Geometry: final body of the model. Coordinates: model frame, mm. Round coordinates to 2 decimals unless told otherwise and drop trailing zeros. Order: outer loops, then holes, each group sorted by start corner. A loop starts at its lowest first (then second) coordinate and runs counter-clockwise, first axis right, second up. Notation, with made-up numbers: M 55,-27.5 L 96,-27.5 A17 ccw 96,-19.5 Z; hole C 78,-3 d8. An arc over 180 degrees is marked long. Return JSON: item names as keys, results as strings. Group by question number.
Q1. Cut plane A-A on z = -46.5. Output: boundary loops of the cut face in (x, y), and give its area (3 significant figures).
Q2. Contact query for flat-ended pins moving along their axis: pin 1 (3 mm diameter, centred on x = -2.5, z = 11, fed in from +Y); pin 2 (3 mm diameter, centred on x = -56, z = -91, fed in from +Y). Output: stop coordinate, or through.
Q3. Cut plane B-B on y = 1.4. Count the separate pieces of the cut face and the enclosed holes in it, and give its area (3 significant figures).
Q4. Ray query, probe 1 along X at (y, z) = (1.7, -58.5); probe 2 along X at (y, z) = (2.4, -9) (3 decimals); probe 3 along Z at (x, y) = (-91, 2.4). Return the intervals inside material, ascending.
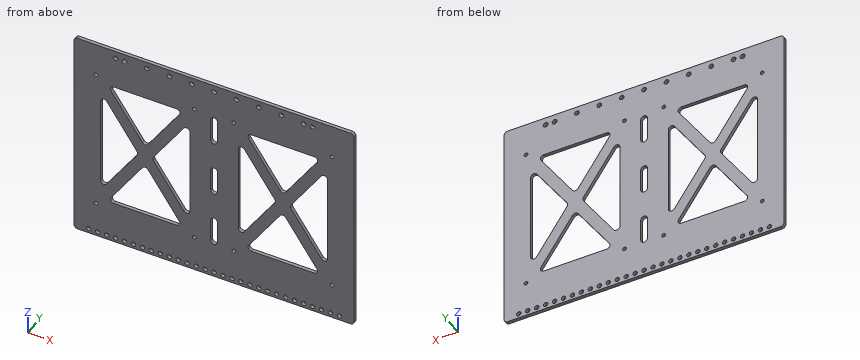
```python
from build123d import *

# Parameters (mm, degrees)
SKETCH_1_W               = 250
SKETCH_1_H               = 190
EXTRUDE_1_DEPTH          = 3
CUT_EXTRUDE_1_DEPTH      = 158.031843904
CUT_EXTRUDE_1_DEPTH_BACK = 158.031843904
SKETCH_3_R               = 2.15
CUT_EXTRUDE_2_DEPTH      = 158.031843904
SKETCH_4_R               = 2.1
CUT_EXTRUDE_3_DEPTH      = 158.031843904
CUT_EXTRUDE_4_DEPTH      = 158.031843904
FILLET_1_R               = 3
CUT_EXTRUDE_5_DEPTH      = 158.031843904


with BuildPart() as part:
    # 草图1 → 凸台-拉伸1 (new body)
    with BuildSketch(Plane(origin=(0, 0, 0), x_dir=(1, 0, 0), z_dir=(0, 1, 0))):
        Rectangle(SKETCH_1_W, SKETCH_1_H)
    extrude(amount=EXTRUDE_1_DEPTH)

    # 草图2 → 切除-拉伸1 (cut, two sides: drawn at the far end of the back side and taken through both)
    with BuildSketch(Plane.XZ.offset(-CUT_EXTRUDE_1_DEPTH_BACK)):
        with BuildLine():
            ThreePointArc((56, -93), (58, -91), (56, -89))
            ThreePointArc((56, -89), (54, -91), (56, -93))
        make_face()
        with BuildLine():
            ThreePointArc((-112, -93), (-110, -91), (-112, -89))
            ThreePointArc((-112, -89), (-114, -91), (-112, -93))
        make_face()
        with BuildLine():
            ThreePointArc((-104, -93), (-102, -91), (-104, -89))
            ThreePointArc((-104, -89), (-106, -91), (-104, -93))
        make_face()
        with BuildLine():
            ThreePointArc((-96, -93), (-94, -91), (-96, -89))
            ThreePointArc((-96, -89), (-98, -91), (-96, -93))
        make_face()
        with BuildLine():
            ThreePointArc((-88, -93), (-86, -91), (-88, -89))
            ThreePointArc((-88, -89), (-90, -91), (-88, -93))
        make_face()
        with BuildLine():
            ThreePointArc((-48, -93), (-46, -91), (-48, -89))
            ThreePointArc((-48, -89), (-50, -91), (-48, -93))
        make_face()
        with BuildLine():
            ThreePointArc((-80, -93), (-78, -91), (-80, -89))
            ThreePointArc((-80, -89), (-82, -91), (-80, -93))
        make_face()
        with BuildLine():
            ThreePointArc((-72, -93), (-70, -91), (-72, -89))
            ThreePointArc((-72, -89), (-74, -91), (-72, -93))
        make_face()
        with BuildLine():
            ThreePointArc((-64, -93), (-62, -91), (-64, -89))
            ThreePointArc((-64, -89), (-66, -91), (-64, -93))
        make_face()
        with BuildLine():
            ThreePointArc((-56, -93), (-54, -91), (-56, -89))
            ThreePointArc((-56, -89), (-58, -91), (-56, -93))
        make_face()
        with BuildLine():
            ThreePointArc((64, -93), (66, -91), (64, -89))
            ThreePointArc((64, -89), (62, -91), (64, -93))
        make_face()
        with BuildLine():
            ThreePointArc((72, -93), (74, -91), (72, -89))
            ThreePointArc((72, -89), (70, -91), (72, -93))
        make_face()
        with BuildLine():
            ThreePointArc((80, -93), (82, -91), (80, -89))
            ThreePointArc((80, -89), (78, -91), (80, -93))
        make_face()
        with BuildLine():
            ThreePointArc((88, -93), (90, -91), (88, -89))
            ThreePointArc((88, -89), (86, -91), (88, -93))
        make_face()
        with BuildLine():
            ThreePointArc((96, -93), (98, -91), (96, -89))
            ThreePointArc((96, -89), (94, -91), (96, -93))
        make_face()
        with BuildLine():
            ThreePointArc((104, -93), (106, -91), (104, -89))
            ThreePointArc((104, -89), (102, -91), (104, -93))
        make_face()
        with BuildLine():
            ThreePointArc((112, -93), (114, -91), (112, -89))
            ThreePointArc((112, -89), (110, -91), (112, -93))
        make_face()
        with BuildLine():
            ThreePointArc((32, -93), (34, -91), (32, -89))
            ThreePointArc((32, -89), (30, -91), (32, -93))
        make_face()
        with BuildLine():
            ThreePointArc((24, -93), (26, -91), (24, -89))
            ThreePointArc((24, -89), (22, -91), (24, -93))
        make_face()
        with BuildLine():
            ThreePointArc((16, -93), (18, -91), (16, -89))
            ThreePointArc((16, -89), (14, -91), (16, -93))
        make_face()
        with BuildLine():
            ThreePointArc((8, -93), (10, -91), (8, -89))
            ThreePointArc((8, -89), (6, -91), (8, -93))
        make_face()
        with BuildLine():
            ThreePointArc((0, -93), (2, -91), (0, -89))
            ThreePointArc((0, -89), (-2, -91), (0, -93))
        make_face()
        with BuildLine():
            ThreePointArc((-8, -93), (-6, -91), (-8, -89))
            ThreePointArc((-8, -89), (-10, -91), (-8, -93))
        make_face()
        with BuildLine():
            ThreePointArc((-16, -93), (-14, -91), (-16, -89))
            ThreePointArc((-16, -89), (-18, -91), (-16, -93))
        make_face()
        with BuildLine():
            ThreePointArc((-24, -93), (-22, -91), (-24, -89))
            ThreePointArc((-24, -89), (-26, -91), (-24, -93))
        make_face()
        with BuildLine():
            ThreePointArc((-32, -93), (-30, -91), (-32, -89))
            ThreePointArc((-32, -89), (-34, -91), (-32, -93))
        make_face()
        with BuildLine():
            ThreePointArc((-40, -93), (-38, -91), (-40, -89))
            ThreePointArc((-40, -89), (-42, -91), (-40, -93))
        make_face()
        with BuildLine():
            ThreePointArc((40, -93), (42, -91), (40, -89))
            ThreePointArc((40, -89), (38, -91), (40, -93))
        make_face()
        with BuildLine():
            ThreePointArc((48, -93), (50, -91), (48, -89))
            ThreePointArc((48, -89), (46, -91), (48, -93))
        make_face()
    extrude(amount=CUT_EXTRUDE_1_DEPTH + CUT_EXTRUDE_1_DEPTH_BACK, mode=Mode.SUBTRACT)

    # 草图3 → 切除-拉伸2 (cut, through all)
    with BuildSketch(Plane(origin=(0, 3, 0), x_dir=(1, 0, 0), z_dir=(0, 1, 0))):
        with Locations(Location((80, -88.135135135, 0), (0, 0, 270))):
            Circle(SKETCH_3_R)
        with Locations(Location((88, -88.135135135, 0), (0, 0, 270))):
            Circle(SKETCH_3_R)
        with Locations(Location((-80, -88.135135135, 0), (0, 0, 270))):
            Circle(SKETCH_3_R)
        with Locations(Location((-88, -88.135135135, 0), (0, 0, 270))):
            Circle(SKETCH_3_R)
        with BuildLine():
            ThreePointArc((105.5, -66.7), (107.2, -65), (105.5, -63.3))
            ThreePointArc((105.5, -63.3), (103.8, -65), (105.5, -66.7))
        make_face()
        with BuildLine():
            ThreePointArc((17.5, -63.3), (15.8, -65), (17.5, -66.7))
            ThreePointArc((17.5, -66.7), (19.2, -65), (17.5, -63.3))
        make_face()
        with BuildLine():
            ThreePointArc((-17.5, -63.3), (-19.2, -65), (-17.5, -66.7))
            ThreePointArc((-17.5, -66.7), (-15.8, -65), (-17.5, -63.3))
        make_face()
        with BuildLine():
            ThreePointArc((-105.5, -66.7), (-103.8, -65), (-105.5, -63.3))
            ThreePointArc((-105.5, -63.3), (-107.2, -65), (-105.5, -66.7))
        make_face()
        with BuildLine():
            ThreePointArc((105.5, 61.3), (107.2, 63), (105.5, 64.7))
            ThreePointArc((105.5, 64.7), (103.8, 63), (105.5, 61.3))
        make_face()
        with BuildLine():
            ThreePointArc((17.5, 64.7), (15.8, 63), (17.5, 61.3))
            ThreePointArc((17.5, 61.3), (19.2, 63), (17.5, 64.7))
        make_face()
        with BuildLine():
            ThreePointArc((-17.5, 61.3), (-15.8, 63), (-17.5, 64.7))
            ThreePointArc((-17.5, 64.7), (-19.2, 63), (-17.5, 61.3))
        make_face()
        with BuildLine():
            ThreePointArc((-105.5, 64.7), (-107.2, 63), (-105.5, 61.3))
            ThreePointArc((-105.5, 61.3), (-103.8, 63), (-105.5, 64.7))
        make_face()
    extrude(amount=-CUT_EXTRUDE_2_DEPTH, mode=Mode.SUBTRACT)

    # 草图4 → 切除-拉伸3 (cut, through all)
    with BuildSketch(Plane(origin=(0, 3, 0), x_dir=(1, 0, 0), z_dir=(0, 1, 0))):
        with Locations(Location((0, -89, 0), (0, 0, 270))):
            Circle(SKETCH_4_R)
        with Locations(Location((20, -89, 0), (0, 0, 270))):
            Circle(SKETCH_4_R)
        with Locations(Location((40, -89, 0), (0, 0, 270))):
            Circle(SKETCH_4_R)
        with Locations(Location((60, -89, 0), (0, 0, 270))):
            Circle(SKETCH_4_R)
        with Locations(Location((-60, -89, 0), (0, 0, 90))):
            Circle(SKETCH_4_R)
        with Locations(Location((-40, -89, 0), (0, 0, 90))):
            Circle(SKETCH_4_R)
        with Locations(Location((-20, -89, 0), (0, 0, 90))):
            Circle(SKETCH_4_R)
    extrude(amount=-CUT_EXTRUDE_3_DEPTH, mode=Mode.SUBTRACT)

    # 草图5 → 切除-拉伸4 (cut, through all)
    with BuildSketch(Plane(origin=(0, 3, 0), x_dir=(1, 0, 0), z_dir=(0, 1, 0))):
        Polygon((-95.30734755, 57), (-61.5, 7.82567629), (-27.69265245, 57), align=None)
        Polygon((-101.375, -50.17432371), (-67.56765245, -1), (-101.375, 48.17432371), align=None)
        Polygon((-95.30734755, -59), (-27.69265245, -59), (-61.5, -9.82567629), align=None)
        Polygon((-55.43234755, -1), (-21.625, -50.17432371), (-21.625, 48.17432371), align=None)
        Polygon((21.625, -50.17432371), (55.43234755, -1), (21.625, 48.17432371), align=None)
        Polygon((61.5, 7.82567629), (95.30734755, 57), (27.69265245, 57), align=None)
        Polygon((101.375, 48.17432371), (67.56765245, -1), (101.375, -50.17432371), align=None)
        Polygon((95.30734755, -59), (61.5, -9.82567629), (27.69265245, -59), align=None)
    extrude(amount=-CUT_EXTRUDE_4_DEPTH, mode=Mode.SUBTRACT)

    # 圆角1
    fillet_1_edges = [part.edges().sort_by_distance(p)[0] for p in [
        (21.625, 1.5, 50.17432371),
        (21.625, 1.5, -48.17432371),
        (55.43234755, 1.5, 1),
        (-55.43234755, 1.5, 1),
        (-21.625, 1.5, -48.17432371),
        (-21.625, 1.5, 50.17432371),
        (-101.375, 1.5, -48.17432371),
        (-67.56765245, 1.5, 1),
        (-101.375, 1.5, 50.17432371),
        (-61.5, 1.5, 9.82567629),
        (-27.69265245, 1.5, 59),
        (-95.30734755, 1.5, 59),
        (27.69265245, 1.5, 59),
        (61.5, 1.5, 9.82567629),
        (95.30734755, 1.5, 59),
        (27.69265245, 1.5, -57),
        (95.30734755, 1.5, -57),
        (61.5, 1.5, -7.82567629),
        (101.375, 1.5, 50.17432371),
        (67.56765245, 1.5, 1),
        (101.375, 1.5, -48.17432371),
        (-95.30734755, 1.5, -57),
        (-27.69265245, 1.5, -57),
        (-61.5, 1.5, -7.82567629),
        (-125, 1.5, -95),
        (-125, 1.5, 95),
        (125, 1.5, 95),
        (125, 1.5, -95),
    ]]
    fillet(fillet_1_edges, radius=FILLET_1_R)

    # 草图6 → 切除-拉伸5 (cut, through all)
    with BuildSketch(Plane(origin=(0, 3, 0), x_dir=(1, 0, 0), z_dir=(0, 1, 0))):
        with BuildLine():
            Line((-3, -10), (-3, 10))
            ThreePointArc((-3, 10), (0, 13), (3, 10))
            Line((3, 10), (3, -10))
            ThreePointArc((3, -10), (0, -13), (-3, -10))
        make_face()
        with BuildLine():
            Line((3, 40), (3, 60))
            ThreePointArc((3, 60), (0, 63), (-3, 60))
            Line((-3, 60), (-3, 40))
            ThreePointArc((-3, 40), (0, 37), (3, 40))
        make_face()
        with BuildLine():
            Line((3, -60), (3, -40))
            ThreePointArc((3, -40), (0, -37), (-3, -40))
            Line((-3, -40), (-3, -60))
            ThreePointArc((-3, -60), (0, -63), (3, -60))
        make_face()
    extrude(amount=-CUT_EXTRUDE_5_DEPTH, mode=Mode.SUBTRACT)


solid = part.part
```
Result sheet:
{
 "1": {"outline": "M -125,0 L -88.09,0 L -88.09,3 L -125,3 Z; M -34.91,0 L -3,0 L -3,3 L -34.91,3 Z; M 3,0 L 34.91,0 L 34.91,3 L 3,3 Z; M 88.09,0 L 125,0 L 125,3 L 88.09,3 Z", "area": "413 mm²"},
 "2": {"pin 1": "stops at y = 3", "pin 2": "passes through"},
 "3": {"separate pieces": "1", "enclosed holes": "59", "area": "33,400 mm²"},
 "4": {"probe 1": "x = -125 to -3, 3 to 125", "probe 2": "x = -125 to -101.375, -74.443 to -48.557, -21.625 to -3, 3 to 21.625, 48.557 to 74.443, 101.375 to 125", "probe 3": "z = -95 to -56.66, -50.73 to -33.08, 35.08 to 52.73, 58.66 to 95"}
}
